Autodesk Inventor part; units mm, degrees
ref_plane "YZ Plane" through (0, 0, 0) normal (1, 0, 0) x (0, 1, 0)
ref_plane "XZ Plane" through (0, 0, 0) normal (0, 1, 0) x (-1, 0, 0)
ref_plane "XY Plane" through (0, 0, 0) normal (0, 0, 1) x (1, 0, 0)
sketch "Sketch1" plane through (0, 0, 0) normal (0, 0, 1) x (1, 0, 0)
  line L0 (-53, 43.3013) -> (103, 43.3013)
  line L1 (-53, 43.3013) -> (-53, -106.6987)
  line L2 (-53, -106.6987) -> (103, -106.6987)
  line L3 (103, -106.6987) -> (103, 43.3013)
  line L4 (0, 0) -> (-53, 0)
  line L5 (0, 0) -> (25, 43.3013)
  line L6 (103, 43.3013) -> (53, 43.3013)
  line L7 (53, 43.3013) -> (53, -6.6987)
  circle A0 centre (53, -6.6987) radius 20
  dimension "d0" = 156
  dimension "d1" = 150
  dimension "d2" = 53
  dimension "d12" = 50
  dimension "d13" = 50
  dimension "d14" = 50
  dimension "d15" = 40
sketch "Sketch2" plane through (0, 0, 0) normal (0, 0, 1) x (1, 0, 0)
  point P0 (0, 0)
extrude "Extrusion1" add sketch "Sketch1" along normal blind 3 contours L0 L5 L4 L1 | A0 | L0 L3 L2 L1 L4 L5
sketch "Sketch3" plane through (103, -106.6987, 0) normal (1, 0, 0) x (0, 0, -1)
  point P0 (0, 106.6987)
sketch "Sketch4" plane through (0, 0, 0) normal (0, 0, 1) x (1, 0, 0)
  point P0 (0, 0)
extrude "Extrusion2" cut sketch "Sketch1" along normal through all contours A0
properties part number "box top"
Check sheet for the modelled part. Datum: model origin and axes. Units: mm. Give positions to 0.01 mm unless a question says otherwise; leave off trailing zeros. Loops run counter-clockwise (first coordinate to the right, second up) from the corner with the lowest first, then second, coordinate; pieces in that order, holes last. Notation, with made-up numbers: M 89,51.25 L 121,51.25 A17 ccw 121,73.25 Z; hole C 48.25,10 d10. An arc over 180 degrees is marked long. Use a Markdown table: item, result. Add a question column.
Q1. Mould release check, pull along Y, two halves, no side actions. Record for faces 1 (the cylindrical face through (72.076, -12.706, 1.479)), 2 (the flat face through (24, -31, 3)): pulls with the +Y half, pulls with the -Y half, needs draft (parallel to the pull), parting line crosses it, or undercut.
Q2. Go/stop test with a flat-tipped pin: pin 1 (8 mm diameter, centred on x = -34.5, y = 13.5, fed in from -Z). Record where the tip stops, or that it passes through.
Q3. Sectioned sample at C-C, the plane y = 8. Record the cut outline in (x, z), then the cut area to 3 significant figures.
Q4. Sectioned sample at A-A, the plane x = 53. Record the cut outline in (y, z), then the cut area to 3 significant figures.
Q5. Sectioned sample at B-B, the plane z = 2.4. Record the cut outline in (x, y), then the cut area to 3 significant figures.
Q6. Scan lines: line 1 along Y through (x, z) = (53, 1.5); line 2 along Y through (x, z) = (54.5, 0.4); line 3 along X through (y, z) = (-21.5, 1.7). Record each from-to range of solid material in increasing order. Write a range as [from, to].
Verdict:
| question | item | result |
|---|---|---|
| 1 | face 1 | undercut |
| 1 | face 2 | needs draft |
| 2 | pin 1 | z = 0 |
| 3 | outline | M -53,0 L 39.44,0 L 39.44,3 L -53,3 Z; M 66.56,0 L 103,0 L 103,3 L 66.56,3 Z |
| 3 | area | 387 mm^2 |
| 4 | outline | M -106.7,0 L -26.7,0 L -26.7,3 L -106.7,3 Z; M 13.3,0 L 43.3,0 L 43.3,3 L 13.3,3 Z |
| 4 | area | 330 mm^2 |
| 5 | outline | M -53,-106.7 L 103,-106.7 L 103,43.3 L -53,43.3 Z; hole C 53,-6.7 d40 |
| 5 | area | 22,100 mm^2 |
| 6 | line 1 | [-106.7, -26.7], [13.3, 43.3] |
| 6 | line 2 | [-106.7, -26.64], [13.24, 43.3] |
| 6 | line 3 | [-53, 39.55], [66.45, 103] |
